from build123d import *

# Parameters (mm, degrees)
EXTRUDE_1_DEPTH    = 5
HOLE_WIZARD_M8_2_D = 6.8


with BuildPart() as part:
    # 草图1 → 凸台-拉伸1 (new body)
    with BuildSketch(Plane.XY):
        with BuildLine():
            Line((-70, 25), (70, 25))
            ThreePointArc((70, 25), (73.535533906, 23.535533906), (75, 20))
            Line((75, 20), (75, -20))
            ThreePointArc((75, -20), (73.535533906, -23.535533906), (70, -25))
            Line((70, -25), (-70, -25))
            ThreePointArc((-70, -25), (-73.535533906, -23.535533906), (-75, -20))
            Line((-75, -20), (-75, 20))
            ThreePointArc((-75, 20), (-73.535533906, 23.535533906), (-70, 25))
        make_face()
    extrude(amount=EXTRUDE_1_DEPTH)

    # M8 螺纹槽口的螺纹槽口钻头2 (through all)
    with Locations(Plane.XY.offset(5)):
        with Locations((-50, 0), (50, 0)):
            Hole(HOLE_WIZARD_M8_2_D / 2)


solid = part.part
Can you work these out from the model? Positions are in its coordinate system, mm. Coordinates: 2 decimals unless noted, no trailing zeros. Order: outer loops, then holes, each group sorted by start corner. A loop starts at its lowest first (then second) coordinate and runs counter-clockwise, first axis right, second up. Notation, with made-up numbers: (52.25, 58) - (106.25, 58) arc R18 cw to (106.25, 75) - close; hole circle Ø11 at (66, 63.5). An arc over 180 degrees is marked (long way). Answer as a JSON object with one key per item and string values. Group by question number.
Q1. Imagine slicing it at B-B (y = 0). Please give me the cut outline in (x, z), and give its area (3 significant figures).
Q2. We'd pull the mould along X, two halves only. Please class faces 1 (the face through (46.86, -1.3, 2.47)), 2 (the face through (1, 0, 0)), 3 (the face through (-53.14, -1.3, 2.47)), 4 (the face through (73, 24, 2)): +X half, -X half, draft (parallel to the pull), parting line (faces both ways), or undercut.
Q3. Imagine slicing it at A-A (x = -50). Please give me the cut outline in (y, z).
Q4. I need wall thicknesses on line 1 (Y direction, x = 50, z = 1.35). Which ranges of the line are inside material? Lowest first, please. Write a range as from..to.
Determined:
{
 "1": {"outline": "(-75, 0) - (-53.4, 0) - (-53.4, 5) - (-75, 5) - close; (-46.6, 0) - (46.6, 0) - (46.6, 5) - (-46.6, 5) - close; (53.4, 0) - (75, 0) - (75, 5) - (53.4, 5) - close", "area": "682 mm2"},
 "2": {"face 1": "undercut", "face 2": "draft", "face 3": "undercut", "face 4": "+X half"},
 "3": {"outline": "(-25, 0) - (-3.4, 0) - (-3.4, 5) - (-25, 5) - close; (3.4, 0) - (25, 0) - (25, 5) - (3.4, 5) - close"},
 "4": {"line 1": "y = -25..-3.4, 3.4..25"}
}
